The drawing under review shows one solid part. Ordinate dimensions are in mm from its lowest x, y, z. A direction names the side the tool comes from. Round coordinates to 2 decimals unless told otherwise and drop trailing zeros. Write each loop counter-clockwise with the first axis right and the second up, starting at its lowest first coordinate (ties: lowest second). Pieces come first, ordered by that corner, then holes. Notation, with made-up numbers: M -36.75,-12 L 5.25,-12 A28 cw 5.25,15 Z; hole C -29.5,83.25 d3. An arc over 180 degrees is marked long. Write item = value, one per line. Start each with the question number.
Item 1: Tool access review of the marked faces 1, 2 and 3: name each direction out of +Z, -Z, +X, -X, +Y, -Y from which nothing blocks a thin tool from reaching the whole face with its end or side.
Item 2: The part is to be moulded in two halves that separate along Y. For the marked faces 4, 5 and 6, say which applies: +Y half, -Y half, draft (parallel to the pull), parting line (faces both ways), or undercut.
Item 3: Take a section at C-C, the plane y = 30. Give the boundary of the cut face in (x, z), plus the area to 3 significant figures.
Item 4: Take a section at B-B, the plane z = 2.4. Give the boundary of the cut face in (x, y).
Item 5: Take a section at D-D, the plane x = 22.5. Give the boundary of the cut face in (y, z) (1 decimal).
Item 6: To check wall thickness, follow line 1 along Y through (x, z) = (18.5, 5.55); line 2 along X through (y, z) = (28, 3.15) (1 decimal); line 3 along X through (y, z) = (29, 2). State the ranges of each line that lie inside material, in increasing order.
Item 7: For pin 1 Ø1.8 at (y, z) = (29.5, 3.5) entering from +X, flat-tipped, find the tip position at first contact; note if it passes through.
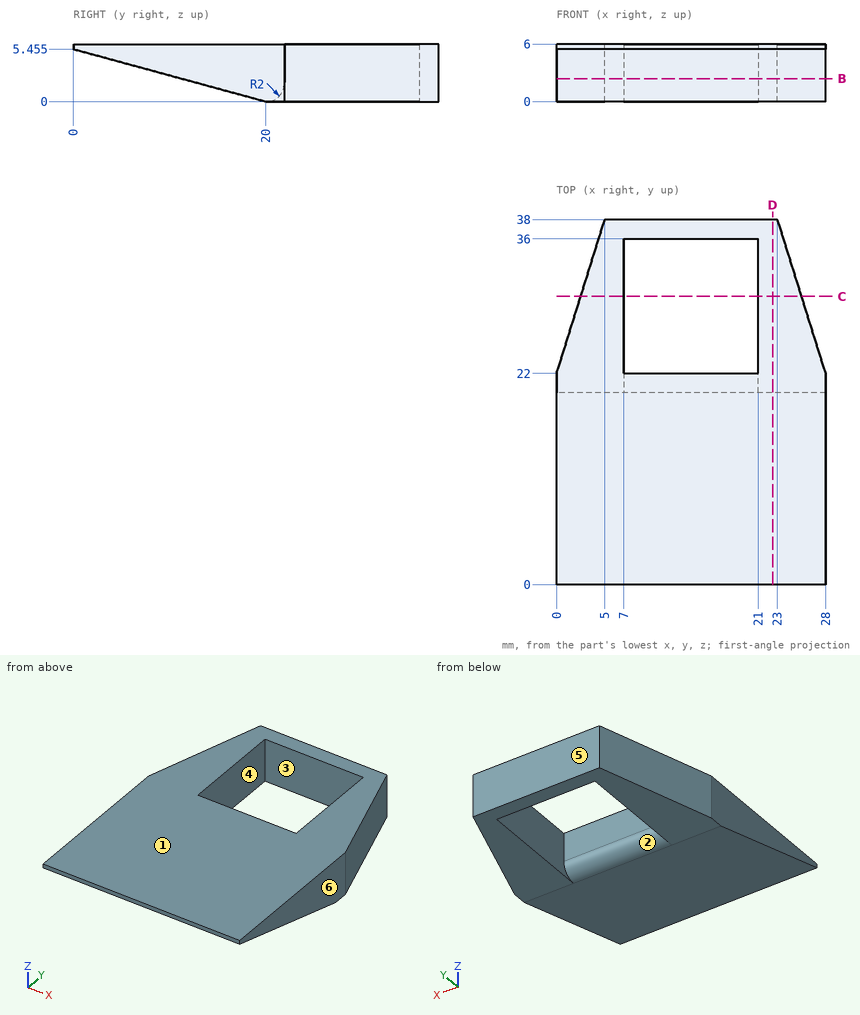
Response values:
q1.face_1 = +Z, +X, -X, +Y, -Y
q1.face_2 = -Z
q1.face_3 = +Z, -Z
q2.face_4 = undercut
q2.face_5 = +Y half
q2.face_6 = draft
q3.outline = M 2.5,0 L 7,0 L 7,6 L 2.5,6 Z; M 21,0 L 25.5,0 L 25.5,6 L 21,6 Z
q3.area = 54.0 mm2
q4.outline = M 0,11.2 L 28,11.2 L 28,22 L 23,38 L 5,38 L 0,22 Z; hole M 7,22 L 21,22 L 21,36 L 7,36 Z
q5.outline = M 0,5.5 L 20,0 L 38,0 L 38,6 L 0,6 Z
q6.line_1 = 0 to 22, 36 to 38
q6.line_2 = 1.9 to 7, 21 to 26.1
q6.line_3 = 2.19 to 7, 21 to 25.81
q7.pin_1 = 25.94
